Source: CAD feature listing. Evaluate the final solid. Frame: model axes, mm. A direction names the side the tool comes from. Round coordinates to 2 decimals unless told otherwise and drop trailing zeros. Write each loop counter-clockwise with the first axis right and the second up, starting at its lowest first coordinate (ties: lowest second). Pieces come first, ordered by that corner, then holes. Notation, with made-up numbers: M -34,-22 L 16,-22 A9 ccw 16,-11 Z; hole C -15.5,-2 d2. An arc over 180 degrees is marked long. Answer in a Markdown table with one row per item.
from build123d import *

# Parameters (mm, degrees)
SKETCH1_W           = 19.05
SKETCH1_H           = 15.875
BOSS_EXTRUDE1_DEPTH = 28.575
BOSS_EXTRUDE2_DEPTH = 9.525


with BuildPart() as part:
    # Sketch1 → Boss-Extrude1 (new body)
    with BuildSketch(Plane(origin=(0, 0, 0), x_dir=(1, 0, 0), z_dir=(0, 1, 0))):
        with Locations((9.525, 7.9375)):
            Rectangle(SKETCH1_W, SKETCH1_H)
    extrude(amount=BOSS_EXTRUDE1_DEPTH)

    # Sketch2 → Boss-Extrude2 (add)
    with BuildSketch(Plane(origin=(0, 28.575, 0), x_dir=(1, 0, 0), z_dir=(0, 1, 0))):
        with BuildLine():
            ThreePointArc((10.31875, 6.35), (9.525, 7.14375), (8.73125, 6.35))
            Line((8.73125, 6.35), (10.31875, 6.35))
        make_face()
        with BuildLine():
            Line((10.31875, 6.35), (8.73125, 6.35))
            ThreePointArc((8.73125, 6.35), (9.525, 5.55625), (10.31875, 6.35))
        make_face()
    extrude(amount=BOSS_EXTRUDE2_DEPTH)


solid = part.part
Q1. Section D-D (z = -3). Return loops of the section in (x, y) (3 decimals).
Solutions:
| item | result |
|---|---|
| outline | M 0,0 L 19.05,0 L 19.05,28.575 L 0,28.575 Z |
Q2. Section A-A (z = -6.35). Return loops of the section in (x, y) (3 decimals).
Solutions:
| item | result |
|---|---|
| outline | M 0,0 L 19.05,0 L 19.05,28.575 L 10.319,28.575 L 10.319,38.1 L 8.731,38.1 L 8.731,28.575 L 0,28.575 Z |
Q3. Section B-B (x = 7). Return loops of the section in (y, z) (3 decimals).
Solutions:
| item | result |
|---|---|
| outline | M 0,-15.875 L 28.575,-15.875 L 28.575,0 L 0,0 Z |
Q4. Material intervals for probe 1 along Y at (x, z) = (16, -7.75) (3 decimals); probe 2 along Z at (x, y) = (9.25, 31.5), sorted ascending.
Solutions:
| item | result |
|---|---|
| probe 1 | y = 0 to 28.575 |
| probe 2 | z = -7.09 to -5.61 |
Q5. Access query for faces 1 (the flat face through (10, 38.1, -6)), 2 (the cylindrical face through (10.1, 33.3, -5.8)). Directions: +Z, -Z, +X, -X, +Y, -Y. A direction counts if a zero-diameter tool reaches every point of the face in a straight line with its end or side. Return the directions, or none.
Solutions:
| item | result |
|---|---|
| face 1 | +Z, -Z, +X, -X, +Y |
| face 2 | +Y |
Q6. Contact query for flat-ended pins moving along their axis: pin 1 Ø3 at (x, z) = (12.5, -13) entering from +Y (3 decimals); pin 2 Ø10 at (x, y) = (6.5, 34) entering from -Z; pin 3 Ø3 at (x, y) = (14, 30.5) entering from -Z. Output: stop coordinate, or through.
Solutions:
| item | result |
|---|---|
| pin 1 | stops at y = 28.575 |
| pin 2 | stops at z = -7.14 |
| pin 3 | passes through |
